The figure shows three views and two pictorial views of one solid part (mm, origin at its lowest corner). Answer the questions. Round coordinates to 2 decimals unless told otherwise and drop trailing zeros. Write each loop counter-clockwise with the first axis right and the second up, starting at its lowest first coordinate (ties: lowest second). Pieces come first, ordered by that corner, then holes.
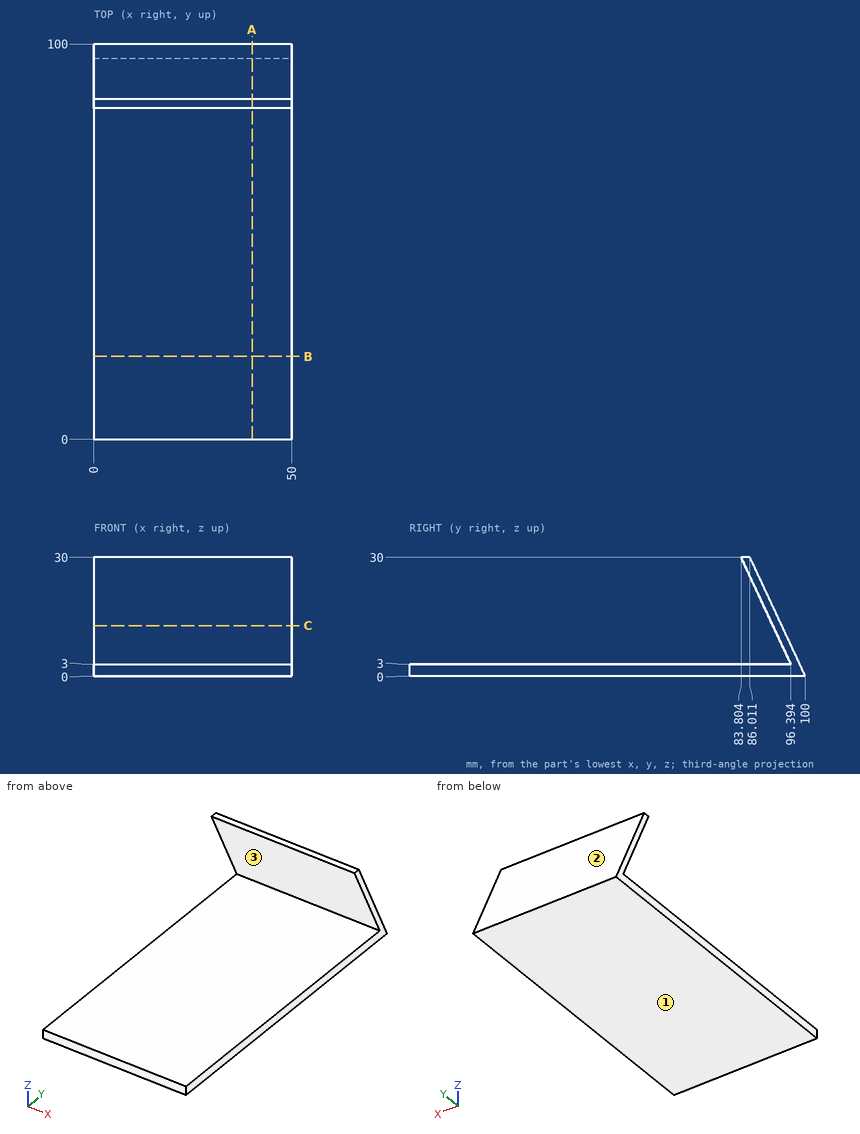
Q1. Flat-ended cylindrical pins translate along their axes: pin 1 Ø10 at (x, z) = (12.5, 7) entering from +Y; pin 2 Ø1 at (x, y) = (32.5, 39.5) entering from +Z. Find the tip coordinate at first contact, or state that the pin passes through.
Verdict:
pin 1: stops at y = 99.07
pin 2: stops at z = 3
Q2. Section A-A (x = 40) is taken. Determine the outline of the cut face in (y, z).
Verdict:
outline: (0, 0) - (100, 0) - (86.01, 30) - (83.8, 30) - (96.39, 3) - (0, 3) - close
Q3. Determine the mould class of the marked faces 1, 2 and 3 for opening direction Z: pulls with the +Z half, pulls with the -Z half, needs draft (parallel to the pull), parting line crosses it, or undercut.
Verdict:
face 1: pulls with the -Z half
face 2: pulls with the +Z half
face 3: undercut
Q4. Straight lines are drawn through the part: probe 1 along Z at (x, y) = (13, 69); probe 2 along Y at (x, z) = (18, 4) (1 decimal); probe 3 along Z at (x, y) = (31, 86.5). For each, find the intervals that lie inside material, in ascending order.
Verdict:
probe 1: z = 0 to 3
probe 2: y = 95.9 to 98.1
probe 3: z = 0 to 3, 24.22 to 28.95
Q5. Section B-B (y = 21) is taken. Determine the outline of the cut face in (x, z).
Verdict:
outline: (0, 0) - (50, 0) - (50, 3) - (0, 3) - close
Q6. Section C-C (z = 12.75) is taken. Determine the outline of the cut face in (x, y) (1 decimal).
Verdict:
outline: (0, 91.8) - (50, 91.8) - (50, 94.1) - (0, 94.1) - close
